Part model, mm, in its own coordinate system. Give positions to 0.01 mm unless a question says otherwise; leave off trailing zeros. Write each loop counter-clockwise with the first axis right and the second up, starting at its lowest first coordinate (ties: lowest second). Pieces come first, ordered by that corner, then holes. Notation, with made-up numbers: M 34.25,86.5 L 51.25,86.5 A24 ccw 51.25,117.5 Z; hole C 84.5,-27 d4. An arc over 180 degrees is marked long. Use a Markdown table: item, result. Add a question column.
from build123d import *

# Parameters (mm, degrees)
CROQUIS1_R              = 75
SALIENTE_EXTRUIR1_DEPTH = 2.5
CROQUIS2_R              = 10
CORTAR_EXTRUIR1_DEPTH   = 5
CROQUIS5_R              = 4.5
CROQUIS3_R              = 2
CORTAR_EXTRUIR4_DEPTH   = 5


with BuildPart() as part:
    # Croquis1 → Saliente-Extruir1 (new, symmetric)
    with BuildSketch(Plane(origin=(0, 0, 0), x_dir=(1, 0, 0), z_dir=(0, 1, 0))):
        with Locations(Location((0, 0, 0), (0, 0, 270))):
            Circle(CROQUIS1_R)
    extrude(amount=SALIENTE_EXTRUIR1_DEPTH, both=True)

    # Croquis2 → Cortar-Extruir1 (cut)
    with BuildSketch(Plane(origin=(0, 2.5, 0), x_dir=(1, 0, 0), z_dir=(0, 1, 0))):
        with Locations(Location((0, 0, 0), (0, 0, 270))):
            Circle(CROQUIS2_R)
    extrude(amount=-CORTAR_EXTRUIR1_DEPTH, mode=Mode.SUBTRACT)

    # Cortar-Barrer1: sweep along a path in Croquis4
    with BuildLine(Plane(origin=(0, 2.5, 0), x_dir=(1, 0, 0), z_dir=(0, 1, 0))) as cortar_barrer1_path:
        CenterArc((0, 0), 64.5, 0, 360)
    # Croquis5 → Cortar-Barrer1 (sweep, cut)
    with BuildSketch(Plane(origin=(0, 0, 0), x_dir=(0, 0, -1), z_dir=(1, 0, 0))):
        with Locations((64.5, 5.5)):
            Circle(CROQUIS5_R)
    sweep(path=cortar_barrer1_path.line, mode=Mode.SUBTRACT)

    # Croquis3 → Cortar-Extruir4 (cut)
    with BuildSketch(Plane(origin=(0, 2.5, 0), x_dir=(1, 0, 0), z_dir=(0, 1, 0))):
        with Locations(Location((-14.5, 10.5, 0), (0, 0, 270))):
            Circle(CROQUIS3_R)
        with Locations(Location((-14.5, 0.5, 0), (0, 0, 270))):
            Circle(CROQUIS3_R)
        with Locations(Location((35.5, 11, 0), (0, 0, 270))):
            Circle(CROQUIS3_R)
        with Locations(Location((35.5, 0.5, 0), (0, 0, 270))):
            Circle(CROQUIS3_R)
    extrude(amount=-CORTAR_EXTRUIR4_DEPTH, mode=Mode.SUBTRACT)


solid = part.part
1. Cut at A-A (x = 0). Write the cut outline in (y, z).
2. Drill centre lines: probe 1 along X at (y, z) = (0.65, -0.5); probe 2 along Z at (x, y) = (28, 2.25); probe 3 along X at (y, z) = (0.9, -10.5). Where is each one in solid material? Low to high. Write a range as [from, to].
3. Cut at C-C (x = 35.5). Give the number of separate pieces and of enclosed holes in the cut face, then the cut area to 3 significant figures.
4. Flat gauge pins, fed straight in: pin 1 (1.5 mm diameter, centred on y = -2, z = -57.5, fed in from -X); pin 2 (23 mm diameter, centred on x = 0, z = 0, fed in from +Y); pin 3 (2 mm diameter, centred on y = 0, z = 43.5, fed in from +X); pin 4 (3 mm diameter, centred on x = 41.5, y = 1, fed in from +Z). Where does each tip first touch, or does it go through?
5. Cut at B-B (y = -0.65). Write the cut outline in (x, z).
6. Mould opens along Z. For faces 1 (the cylindrical face through (33.548, 0.035, -11.434)), 2 (the flat face through (1, 2.5, 13)), 3 (the cylindrical face through (-45.636, 0.035, -59.517)) say: released by +Z, released by -Z, zero draft, split by the parting line, or undercut.
A:
| question | item | result |
|---|---|---|
| 1 | outline | M -2.5,-75 L 2.5,-75 L 2.5,-67.85 A4.5 cw 2.5,-61.15 L 2.5,-10 L -2.5,-10 Z; M -2.5,10 L 2.5,10 L 2.5,61.15 A4.5 cw 2.5,67.85 L 2.5,75 L -2.5,75 Z |
| 2 | probe 1 | x = [-75, -16.5], [-12.5, -9.99], [9.99, 33.5], [37.5, 75] |
| 2 | probe 2 | z = [-69.58, -61.54], [-54.63, 54.63], [61.54, 69.58] |
| 2 | probe 3 | x = [-74.26, -16.5], [-12.5, 33.56], [37.44, 74.26] |
| 3 | separate pieces | 3 |
| 3 | enclosed holes | 0 |
| 3 | area | 604 mm² |
| 4 | pin 1 | stops at x = -49.04 |
| 4 | pin 2 | stops at y = 2.5 |
| 4 | pin 3 | stops at x = 61.8 |
| 4 | pin 4 | stops at z = 63.44 |
| 5 | outline | C 0,0 d150; hole C -14.5,-10.5 d4; hole C -14.5,-0.5 d4; hole C 0,0 d20; hole C 35.5,-11 d4; hole C 35.5,-0.5 d4 |
| 6 | face 1 | undercut |
| 6 | face 2 | zero draft |
| 6 | face 3 | split by the parting line |
